from build123d import *

# Parameters (mm, degrees)
BOSS_EXTRUDE1_DEPTH = 9
CUT_EXTRUDE2_REACH  = 95.842
SKETCH5_W           = 20
SKETCH5_H           = 32
SKETCH5_W_2         = 7.75
CUT_EXTRUDE3_DEPTH  = 10
FILLET1_R           = 5
CUT_EXTRUDE4_DEPTH  = 4
CHAMFER1_SIZE       = 9
CHAMFER1_SIZE_2     = 4.196768923
FILLET2_R           = 10
CUT_EXTRUDE5_REACH  = 95.842
SKETCH7_W           = 5
SKETCH7_H           = 33.085129134
SKETCH7_H_2         = 33.745309592


with BuildPart() as part:
    # Sketch1 → Boss-Extrude1 (new body)
    with BuildSketch(Plane(origin=(0, 0, 0), x_dir=(1, 0, 0), z_dir=(0, 1, 0))):
        Polygon((0, 0), (0, 55), (75.5, 55), (75.5, 0), (37.75, 13.739876344), align=None)
    extrude(amount=BOSS_EXTRUDE1_DEPTH)

    # Sketch4 → Cut-Extrude2 (cut, up to next)
    with BuildSketch(Plane(origin=(0, 9, 0), x_dir=(1, 0, 0), z_dir=(0, 1, 0)), mode=Mode.PRIVATE) as cut_extrude2_sk1:
        with BuildLine():
            Line((19.25, 48), (19.25, 23))
            ThreePointArc((19.25, 23), (17.75, 21.5), (16.25, 23))
            Line((16.25, 23), (16.25, 48))
            ThreePointArc((16.25, 48), (17.75, 49.5), (19.25, 48))
        make_face()
    cut_extrude2_tool1 = extrude(cut_extrude2_sk1.sketch, amount=-CUT_EXTRUDE2_REACH, mode=Mode.PRIVATE) & part.part
    # Sketch4 → Cut-Extrude2 (cut, up to next)
    with BuildSketch(Plane(origin=(0, 9, 0), x_dir=(1, 0, 0), z_dir=(0, 1, 0)), mode=Mode.PRIVATE) as cut_extrude2_sk2:
        with BuildLine():
            Line((59.25, 48), (59.25, 23))
            ThreePointArc((59.25, 23), (57.75, 21.5), (56.25, 23))
            Line((56.25, 23), (56.25, 48))
            ThreePointArc((56.25, 48), (57.75, 49.5), (59.25, 48))
        make_face()
    cut_extrude2_tool2 = extrude(cut_extrude2_sk2.sketch, amount=-CUT_EXTRUDE2_REACH, mode=Mode.PRIVATE) & part.part
    add(cut_extrude2_tool1.solids().sort_by_distance((17.75, 9, -35.5))[0], mode=Mode.SUBTRACT)
    add(cut_extrude2_tool2.solids().sort_by_distance((57.75, 9, -35.5))[0], mode=Mode.SUBTRACT)

    # Sketch5 → Cut-Extrude3 (cut)
    with BuildSketch(Plane(origin=(0, 9, 0), x_dir=(1, 0, 0), z_dir=(0, 1, 0))):
        with Locations((37.75, 39)):
            Rectangle(SKETCH5_W, SKETCH5_H)
        with Locations((71.625, 39)):
            Rectangle(SKETCH5_W_2, SKETCH5_H)
        with Locations((3.875, 39)):
            Rectangle(SKETCH5_W_2, SKETCH5_H)
    extrude(amount=-CUT_EXTRUDE3_DEPTH, mode=Mode.SUBTRACT)

    # Fillet1
    fillet1_edges = [part.edges().sort_by_distance(p)[0] for p in [
        (27.75, 4.5, -23),
        (47.75, 4.5, -23),
        (7.75, 4.5, -23),
        (67.75, 4.5, -23),
    ]]
    fillet(fillet1_edges, radius=FILLET1_R)

    # Sketch6 → Cut-Extrude4 (cut)
    with BuildSketch(Plane(origin=(0, 9, 0), x_dir=(1, 0, 0), z_dir=(0, 1, 0))):
        with BuildLine():
            Line((20.55, 48), (20.55, 23))
            ThreePointArc((20.55, 23), (17.75, 20.2), (14.95, 23))
            Line((14.95, 23), (14.95, 48))
            ThreePointArc((14.95, 48), (17.75, 50.8), (20.55, 48))
        make_face()
        with BuildLine():
            Line((60.55, 48), (60.55, 23))
            ThreePointArc((60.55, 23), (57.75, 20.2), (54.95, 23))
            Line((54.95, 23), (54.95, 48))
            ThreePointArc((54.95, 48), (57.75, 50.8), (60.55, 48))
        make_face()
    extrude(amount=-CUT_EXTRUDE4_DEPTH, mode=Mode.SUBTRACT)

    # Chamfer1
    # the kernel refuses this chamfer: 9, 4.196768923 mm, written as the material it takes off along each edge
    with BuildSketch(Plane(origin=(97.41248478, 9, 7.975492219), x_dir=(-0.005578746693930982, -0.9998669641130703, 0.015327480570432298), z_dir=(-0.939692620785907, 0, -0.3420201433256727))) as chamfer1_piece_1_section:
        Polygon((CHAMFER1_SIZE * 0.999866964113, -CHAMFER1_SIZE * 0.0163111641311), (-CHAMFER1_SIZE_2 * 0.0163111641326, -CHAMFER1_SIZE_2 * 0.999866964207), (0, 0), align=None)
    chamfer1_piece_1 = extrude(amount=86.810269397, mode=Mode.PRIVATE)
    chamfer1_piece_1 = split(chamfer1_piece_1, bisect_by=Plane(origin=(61.945555659, 5.929396418, -22.546338405), z_dir=(0.3420201433256727, 0, 0.939692620785907)), keep=Keep.TOP, mode=Mode.PRIVATE)
    add(chamfer1_piece_1, mode=Mode.SUBTRACT)
    with BuildSketch(Plane(origin=(59.66248478, 9, -21.715368562), x_dir=(0.0055787466939309265, -0.9998669641130703, 0.015327480570432147), z_dir=(-0.939692620785907, 0, 0.3420201433256727))) as chamfer1_piece_2_section:
        Polygon((CHAMFER1_SIZE * 0.999866964113, -CHAMFER1_SIZE * 0.0163111641311), (-CHAMFER1_SIZE_2 * 0.0163111641326, -CHAMFER1_SIZE_2 * 0.999866964207), (0, 0), align=None)
    chamfer1_piece_2 = extrude(amount=86.810269397, mode=Mode.PRIVATE)
    chamfer1_piece_2 = split(chamfer1_piece_2, bisect_by=Plane(origin=(13.554444341, 5.929396418, -22.546338405), z_dir=(-0.3420201433256727, 0, 0.939692620785907)), keep=Keep.TOP, mode=Mode.PRIVATE)
    add(chamfer1_piece_2, mode=Mode.SUBTRACT)
    with BuildSketch(Plane(origin=(97.41248478, 9, 7.975492219), x_dir=(-0.005578746693930982, -0.9998669641130703, 0.015327480570432298), z_dir=(-0.939692620785907, 0, -0.3420201433256727))) as chamfer1_piece_3a_section:
        Polygon((CHAMFER1_SIZE * 0.999866964113, -CHAMFER1_SIZE * 0.0163111641311), (-CHAMFER1_SIZE_2 * 0.0163111641326, -CHAMFER1_SIZE_2 * 0.999866964207), (0, 0), align=None)
    chamfer1_piece_3a = extrude(amount=86.810269397, mode=Mode.PRIVATE)
    chamfer1_piece_3a = split(chamfer1_piece_3a, bisect_by=Plane(origin=(30.782637317, 6.02174195, -11.203963716), z_dir=(-0.3420201433256727, 0, -0.939692620785907)), keep=Keep.TOP, mode=Mode.PRIVATE)
    with BuildSketch(Plane(origin=(59.66248478, 9, -21.715368562), x_dir=(0.0055787466939309265, -0.9998669641130703, 0.015327480570432147), z_dir=(-0.939692620785907, 0, 0.3420201433256727))) as chamfer1_piece_3b_section:
        Polygon((CHAMFER1_SIZE * 0.999866964113, -CHAMFER1_SIZE * 0.0163111641311), (-CHAMFER1_SIZE_2 * 0.0163111641326, -CHAMFER1_SIZE_2 * 0.999866964207), (0, 0), align=None)
    chamfer1_piece_3b = extrude(amount=86.810269397, mode=Mode.PRIVATE)
    chamfer1_piece_3b = split(chamfer1_piece_3b, bisect_by=Plane(origin=(44.717362683, 6.02174195, -11.203963716), z_dir=(0.3420201433256727, 0, -0.939692620785907)), keep=Keep.TOP, mode=Mode.PRIVATE)
    chamfer1_piece_3 = chamfer1_piece_3a & chamfer1_piece_3b
    add(chamfer1_piece_3, mode=Mode.SUBTRACT)

    # Fillet2
    fillet2_edges = [part.edges().sort_by_distance(p)[0] for p in [
        (37.75, 4.5, -15.972930446),
    ]]
    fillet(fillet2_edges, radius=FILLET2_R)

    # Sketch7 → Cut-Extrude5 (cut, up to next)
    with BuildSketch(Plane(origin=(0, 9, 0), x_dir=(1, 0, 0), z_dir=(0, 1, 0)), mode=Mode.PRIVATE) as cut_extrude5_sk1:
        with Locations((2.5, 16.542564567)):
            Rectangle(SKETCH7_W, SKETCH7_H)
    cut_extrude5_tool1 = extrude(cut_extrude5_sk1.sketch, amount=-CUT_EXTRUDE5_REACH, mode=Mode.PRIVATE) & part.part
    # Sketch7 → Cut-Extrude5 (cut, up to next)
    with BuildSketch(Plane(origin=(0, 9, 0), x_dir=(1, 0, 0), z_dir=(0, 1, 0)), mode=Mode.PRIVATE) as cut_extrude5_sk2:
        with Locations((73, 16.872654796)):
            Rectangle(SKETCH7_W, SKETCH7_H_2)
    cut_extrude5_tool2 = extrude(cut_extrude5_sk2.sketch, amount=-CUT_EXTRUDE5_REACH, mode=Mode.PRIVATE) & part.part
    add(cut_extrude5_tool1.solids().sort_by_distance((2.5, 9, -16.542565))[0], mode=Mode.SUBTRACT)
    add(cut_extrude5_tool2.solids().sort_by_distance((73, 9, -16.872655))[0], mode=Mode.SUBTRACT)


solid = part.part
For this review, take the finished solid that the model builds, in its own axes (mm). A direction names the side the tool comes from. Round coordinates to 2 decimals unless told otherwise and drop trailing zeros. Loops run counter-clockwise (first coordinate to the right, second up) from the corner with the lowest first, then second, coordinate; pieces in that order, holes last. Notation, with made-up numbers: (-10, 70) - (28, 70) arc R37 ccw to (28, 109) - close; hole circle Ø9 at (73.25, 71.5). An arc over 180 degrees is marked (long way). Put each result on its own line as item: value. Start each with the question number.
1. Consider section C-C on z = -9. State the section outline as (x, y) points, plus the area to 3 significant figures.
2. For faces 1 (the flat face through (56.25, 3, -35)), 2 (the cylindrical face through (57.7, 7, -50.8)), 3 (the flat face through (7.75, 5, -41)), 4 (the flat face through (27.75, 5, -41)), 5 (the flat face through (45, 0, -23)), list the 3-axis set-ups (+Z, -Z, +X, -X, +Y, -Y) from which the entire face can be reached by the end or side of a thin tool; tool diameter is ignored.
3. Insertion check: P1, Ø1.7, axis at x = 17, z = -43, coming from the +Y side; P2, Ø5, axis at x = 24, y = 1.5, coming from the +Z side; P3, Ø2.5, axis at y = 3, z = -41, coming from the +X side. Each pin has a flat end and moves straight along its axis. Give the tip position at first contact, or say it passes through.
4. Mouldability with a two-part tool opening along Z and no side actions: class faces 6 (the flat face through (59.25, 3, -36)), 7 (the cylindrical face through (46.32, 4.44, -24.5)), 8 (the flat face through (70.5, 5, -13)) as +Z half, -Z half, draft (parallel to the pull), parting line (faces both ways), or undercut.
5. Consider section B-B on x = 58.5. State the section outline as (y, z) points, plus the area to 3 significant figures.
6. Consider section A-A on z = -25. State the section outline as (x, y) points, plus the area to 3 significant figures.
7. For probe 1 along X at (y, z) = (6, -38); probe 2 along X at (y, z) = (3.75, -35); probe 3 along X at (y, z) = (1.75, -52.5), list the stretches that pass through material, from the lowest coordinate up. Write a range as [from, to].
8. Consider section D-D on z = -44.5. State the section outline as (x, y) points.
Result sheet:
1. outline: (5, 0) - (24.73, 0) - (12.46, 9) - (5, 9) - close; (50.77, 0) - (70.5, 0) - (70.5, 9) - (63.04, 9) - close
1. area: 245 mm^2
2. face 1: +Y, -Y
2. face 2: +Y
2. face 3: -Z, -X, +Y, -Y
2. face 4: -Z, +Y, -Y
2. face 5: +Z, -Z, +X, -X, -Y
3. P1: y = 5
3. P2: z = -8.01
3. P3: x = 67.75
4. face 6: undercut
4. face 7: -Z half
4. face 8: draft
5. outline: (0, -55) - (9, -55) - (9, -50.7) - (5, -50.7) - (5, -49.3) - (0, -49.3) - close; (0, -21.7) - (5, -21.7) - (5, -20.3) - (9, -20.3) - (9, -10.65) - (0, -6.19) - close
5. area: 160 mm^2
6. outline: (6.75, 0) - (16.25, 0) - (16.25, 5) - (14.95, 5) - (14.95, 9) - (6.75, 9) - close; (19.25, 0) - (28.75, 0) - (28.75, 9) - (20.55, 9) - (20.55, 5) - (19.25, 5) - close; (46.75, 0) - (56.25, 0) - (56.25, 5) - (54.95, 5) - (54.95, 9) - (46.75, 9) - close; (59.25, 0) - (68.75, 0) - (68.75, 9) - (60.55, 9) - (60.55, 5) - (59.25, 5) - close
6. area: 321 mm^2
7. probe 1: [7.75, 14.95], [20.55, 27.75], [47.75, 54.95], [60.55, 67.75]
7. probe 2: [7.75, 16.25], [19.25, 27.75], [47.75, 56.25], [59.25, 67.75]
7. probe 3: [7.75, 27.75], [47.75, 67.75]
8. outline: (7.75, 0) - (16.25, 0) - (16.25, 5) - (14.95, 5) - (14.95, 9) - (7.75, 9) - close; (19.25, 0) - (27.75, 0) - (27.75, 9) - (20.55, 9) - (20.55, 5) - (19.25, 5) - close; (47.75, 0) - (56.25, 0) - (56.25, 5) - (54.95, 5) - (54.95, 9) - (47.75, 9) - close; (59.25, 0) - (67.75, 0) - (67.75, 9) - (60.55, 9) - (60.55, 5) - (59.25, 5) - close
